```python
from build123d import *

# Parameters (mm, degrees)
SKETCH1_W           = 101.6
SKETCH1_H           = 95.25
BOSS_EXTRUDE1_DEPTH = 6.35
SKETCH2_W           = 12.7
SKETCH2_H           = 6.35
SKETCH2_R           = 1.651
SKETCH2_W_2         = 6.35
SKETCH2_H_2         = 12.7
BOSS_EXTRUDE2_DEPTH = 6.35
SKETCH5_R           = 2.4257
CUT_EXTRUDE1_DEPTH  = 80.746567925
FILLET1_R           = 5.08
FILLET2_R           = 1.27


with BuildPart() as part:
    # Sketch1 → Boss-Extrude1 (new body)
    with BuildSketch(Plane.XY):
        with Locations((0, -7.629593436)):
            Rectangle(SKETCH1_W, SKETCH1_H)
    extrude(amount=BOSS_EXTRUDE1_DEPTH)

    # Sketch2 → Boss-Extrude2 (add)
    # profile 1 of 6: a face of its own
    with BuildSketch(Plane.XY.offset(6.35)):
        with Locations((-25.4, 43.170406564)):
            Rectangle(SKETCH2_W, SKETCH2_H)
        with Locations((-25.4, 43.170406564)):
            Circle(SKETCH2_R, mode=Mode.SUBTRACT)
    # profile 2 of 6: a face of its own
    with BuildSketch(Plane.XY.offset(6.35)):
        with Locations((25.4, 43.170406564)):
            Rectangle(SKETCH2_W, SKETCH2_H)
        with Locations((25.4, 43.170406564)):
            Circle(SKETCH2_R, mode=Mode.SUBTRACT)
    # profile 3 of 6: a face of its own
    with BuildSketch(Plane.XY.offset(6.35)):
        with Locations((53.975, 14.595406564)):
            Rectangle(SKETCH2_W_2, SKETCH2_H_2)
        with Locations((53.975, 14.595406564)):
            Circle(SKETCH2_R, mode=Mode.SUBTRACT)
    # profile 4 of 6: a face of its own
    with BuildSketch(Plane.XY.offset(6.35)):
        with Locations((-53.975, 14.595406564)):
            Rectangle(SKETCH2_W_2, SKETCH2_H_2)
        with Locations((-53.975, 14.595406564)):
            Circle(SKETCH2_R, mode=Mode.SUBTRACT)
    # profile 5 of 6: a face of its own
    with BuildSketch(Plane.XY.offset(6.35)):
        with Locations((-53.975, -23.504593436)):
            Rectangle(SKETCH2_W_2, SKETCH2_H_2)
        with Locations((-53.975, -23.504593436)):
            Circle(SKETCH2_R, mode=Mode.SUBTRACT)
    # profile 6 of 6: a face of its own
    with BuildSketch(Plane.XY.offset(6.35)):
        with Locations((53.975, -23.504593436)):
            Rectangle(SKETCH2_W_2, SKETCH2_H_2)
        with Locations((53.975, -23.504593436)):
            Circle(SKETCH2_R, mode=Mode.SUBTRACT)
    extrude(amount=-BOSS_EXTRUDE2_DEPTH)

    # Sketch5 → Cut-Extrude1 (cut, through all)
    with BuildSketch(Plane.XY.offset(6.35)):
        with Locations((-25, 17.370406564)):
            Circle(SKETCH5_R)
        with Locations((25, 17.370406564)):
            Circle(SKETCH5_R)
        with Locations((25, -32.629593436)):
            Circle(SKETCH5_R)
        with Locations((-25, -32.629593436)):
            Circle(SKETCH5_R)
        with BuildLine():
            Line((-24.128510609, -27.305247108), (-15.606604031, -17.040561021))
            ThreePointArc((-15.606604031, -17.040561021), (-16.83342633, -0.646173195), (-4.361627061, 10.065281801))
            Line((-4.361627061, 10.065281801), (-8.664406389, 21.887070846))
            Line((-8.664406389, 21.887070846), (-14.2875, 21.887070846))
            Line((-14.2875, 21.887070846), (-29.516664282, 6.657906564))
            Line((-29.516664282, 6.657906564), (-29.516664282, -21.917093436))
            Line((-29.516664282, -21.917093436), (-24.128510609, -27.305247108))
        make_face()
        with BuildLine():
            Line((-21.317277104, -30.116480614), (-13.135965935, -20.262043681))
            ThreePointArc((-13.135965935, -20.262043681), (0.990969666, -25.827131164), (14.430051116, -18.760901761))
            Line((14.430051116, -18.760901761), (29.516664282, -21.42107871))
            Line((29.516664282, -21.42107871), (29.516664282, -21.917093436))
            Line((29.516664282, -21.917093436), (14.2875, -37.146257718))
            Line((14.2875, -37.146257718), (-14.2875, -37.146257718))
            Line((-14.2875, -37.146257718), (-21.317277104, -30.116480614))
        make_face()
        with BuildLine():
            Line((29.516664282, -12.834177729), (17.947628895, -10.79424465))
            ThreePointArc((17.947628895, -10.79424465), (13.960776954, 4.084889357), (0, 10.594906564))
            Line((0, 10.594906564), (-4.110011679, 21.887070846))
            Line((-4.110011679, 21.887070846), (14.2875, 21.887070846))
            Line((14.2875, 21.887070846), (29.516664282, 6.657906564))
            Line((29.516664282, 6.657906564), (29.516664282, -12.834177729))
        make_face()
    extrude(amount=-CUT_EXTRUDE1_DEPTH, mode=Mode.SUBTRACT)

    # Fillet1
    fillet1_edges = [part.edges().sort_by_distance(p)[0] for p in [
        (-29.516664282, 6.657906564, 3.175),
        (-14.2875, 21.887070846, 3.175),
        (-29.516664282, -21.917093436, 3.175),
        (14.2875, -37.146257718, 3.175),
        (-14.2875, -37.146257718, 3.175),
        (14.2875, 21.887070846, 3.175),
        (29.516664282, 6.657906564, 3.175),
    ]]
    fillet(fillet1_edges, radius=FILLET1_R)

    # Fillet2
    fillet2_edges = [part.edges().sort_by_distance(p)[0] for p in [
        (-4.361627061, 10.065281801, 3.175),
        (-15.606604031, -17.040561021, 3.175),
        (-13.135965935, -20.262043681, 3.175),
        (14.430051116, -18.760901761, 3.175),
        (17.947628895, -10.79424465, 3.175),
        (0, 10.594906564, 3.175),
    ]]
    fillet(fillet2_edges, radius=FILLET2_R)


solid = part.part
```
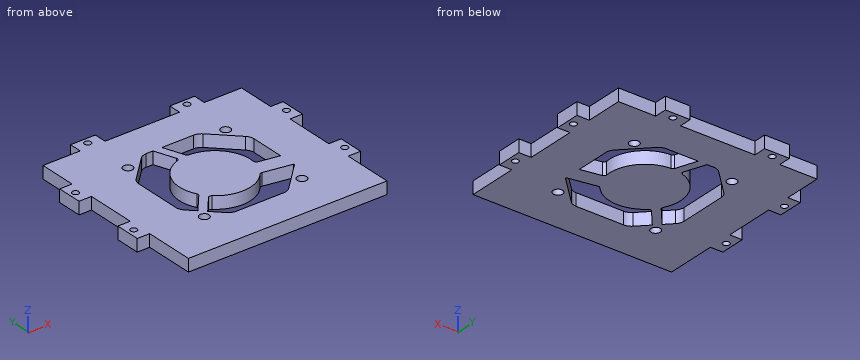
Could you check a few things on this model? Use its own coordinates, in mm. Coordinates: 2 decimals unless noted, no trailing zeros. Write each loop counter-clockwise with the first axis right and the second up, starting at its lowest first coordinate (ties: lowest second). Pieces come first, ordered by that corner, then holes. Notation, with made-up numbers: (88.5, 65) - (104.5, 65) arc R24 ccw to (104.5, 95) - close; hole circle Ø3 at (19.5, 59.5). An arc over 180 degrees is marked (long way). Use a Markdown table: item, result.
Q1. I'm going to push flat-ended pins straight in: pin 1 Ø2 at (y, z) = (-11.5, 3.5) entering from +X; pin 2 Ø1 at (x, y) = (-35, -41) entering from -Z; pin 3 Ø1.9 at (y, z) = (42.5, 4.5) entering from -X; pin 4 Ø2.5 at (x, y) = (25.4, 43.17) entering from +Z. Where does each tip first touch, or does it pass through?
Geometry check:
| item | result |
|---|---|
| pin 1 | stops at x = 50.8 |
| pin 2 | stops at z = 0 |
| pin 3 | stops at x = -31.75 |
| pin 4 | passes through |
Q2. Imagine slicing it at C-C (y = -46). List the corners of the cut face in (x, z) for me, and give its area (3 significant figures).
Geometry check:
| item | result |
|---|---|
| outline | (-50.8, 0) - (50.8, 0) - (50.8, 6.35) - (-50.8, 6.35) - close |
| area | 645 mm2 |
Q3. Imagine slicing it at D-D (x = 46). List the corners of the cut face in (y, z) for me, and give its area (3 significant figures).
Geometry check:
| item | result |
|---|---|
| outline | (-55.25, 0) - (40, 0) - (40, 6.35) - (-55.25, 6.35) - close |
| area | 605 mm2 |
Q4. Imagine slicing it at A-A (x = 25.4). List the corners of the cut face in (y, z) for me.
Geometry check:
| item | result |
|---|---|
| outline | (-55.25, 0) - (-35.02, 0) - (-35.02, 6.35) - (-55.25, 6.35) - close; (-30.24, 0) - (-26.03, 0) - (-26.03, 6.35) - (-30.24, 6.35) - close; (-20.7, 0) - (-12.11, 0) - (-12.11, 6.35) - (-20.7, 6.35) - close; (10.77, 0) - (14.98, 0) - (14.98, 6.35) - (10.77, 6.35) - close; (19.76, 0) - (41.52, 0) - (41.52, 6.35) - (19.76, 6.35) - close; (44.82, 0) - (46.35, 0) - (46.35, 6.35) - (44.82, 6.35) - close |
Q5. Imagine slicing it at B-B (x = -25.4). List the corners of the cut face in (y, z) for me, and give its area (3 significant figures).
Geometry check:
| item | result |
|---|---|
| outline | (-55.25, 0) - (-35.02, 0) - (-35.02, 6.35) - (-55.25, 6.35) - close; (-30.24, 0) - (-26.03, 0) - (-26.03, 6.35) - (-30.24, 6.35) - close; (10.77, 0) - (14.98, 0) - (14.98, 6.35) - (10.77, 6.35) - close; (19.76, 0) - (41.52, 0) - (41.52, 6.35) - (19.76, 6.35) - close; (44.82, 0) - (46.35, 0) - (46.35, 6.35) - (44.82, 6.35) - close |
| area | 330 mm2 |
Q6. Please list where these lines run through material, in increasing order: L1, parallel to Y at x = -51, z = 2; L2, parallel to Y at x = 29, z = 1.5; L3, parallel to X at y = -10, z = 1.
Geometry check:
| item | result |
|---|---|
| L1 | y = -29.85 to -17.15, 8.25 to 20.95 |
| L2 | y = -55.25 to -22.43, -21.33 to -12.74, 6.79 to 46.35 |
| L3 | x = -50.8 to -29.52, -18.07 to 18.13, 29.52 to 50.8 |
